Build history of the part. All positions in model axes, mm. Round coordinates to 2 decimals unless told otherwise and drop trailing zeros. Order: outer loops, then holes, each group sorted by start corner. A loop starts at its lowest first (then second) coordinate and runs counter-clockwise, first axis right, second up. Notation, with made-up numbers: (75, 55) -> (110, 55) arc R27 cw to (110, 82) -> close; hole circle Ø8 at (-2.75, 86.25). An arc over 180 degrees is marked (long way). Answer as a JSON object with one key per item and string values.
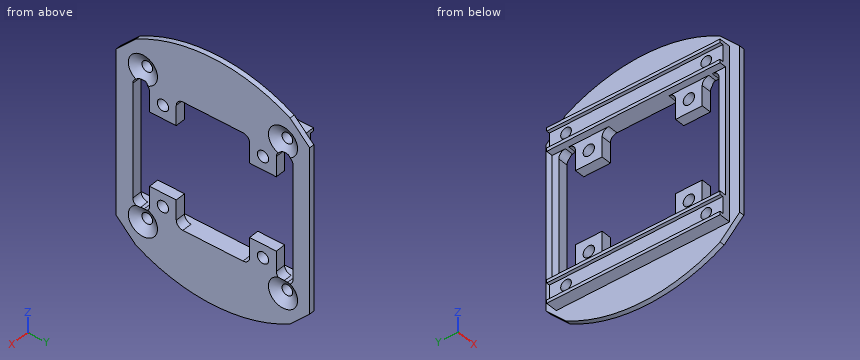
from build123d import *

# Parameters (mm, degrees)
SKETCH_1_W                  = 58
SKETCH_1_H                  = 58
SKETCH_1_R                  = 1.7
EXTRUDE_1_DEPTH             = 5
SKETCH_2_W                  = 58
SKETCH_2_H                  = 58
SKETCH_2_W_2                = 52
SKETCH_2_H_2                = 52
CUT_EXTRUDE_1_DEPTH         = 3.5
SKETCH_3_W                  = 38
SKETCH_3_H                  = 52
CUT_EXTRUDE_2_DEPTH         = 2
SKETCH_4_W                  = 5
SKETCH_4_H                  = 52
CUT_EXTRUDE_3_DEPTH         = 1
SKETCH_8_R                  = 1.6
CUT_EXTRUDE_4_DEPTH         = 2.4
PATTERN_LINEAR_1_COUNT      = 2
PATTERN_LINEAR_1_PITCH      = 45
PATTERN_LINEAR_1_COUNT_DIR2 = 2
PATTERN_LINEAR_1_PITCH_DIR2 = 42
EXTRUDE_2_DEPTH             = 1.5
SKETCH_12_R                 = 63.004873171
CUT_EXTRUDE_6_DEPTH         = 1.5
CHAMFER_2_SIZE              = 2
CHAMFER_3_SIZE              = 2
CHAMFER_5_SIZE              = 2
CHAMFER_6_SIZE              = 2


with BuildPart() as part:
    # 草图1 → 凸台-拉伸1 (new body)
    with BuildSketch(Plane(origin=(0, 0, 0), x_dir=(0, 0, -1), z_dir=(1, 0, 0))):
        Rectangle(SKETCH_1_W, SKETCH_1_H)
        with Locations((15, 15)):
            Circle(SKETCH_1_R, mode=Mode.SUBTRACT)
        with Locations(Location((-15, 15, 0), (0, 0, 180))):
            Circle(SKETCH_1_R, mode=Mode.SUBTRACT)
        with Locations((-15, -15)):
            Circle(SKETCH_1_R, mode=Mode.SUBTRACT)
        with Locations(Location((15, -15, 0), (0, 0, 180))):
            Circle(SKETCH_1_R, mode=Mode.SUBTRACT)
        with BuildLine():
            Line((-17, 24), (17, 24))
            ThreePointArc((17, 24), (18.414213562, 23.414213562), (19, 22))
            Line((19, 22), (19, 21))
            ThreePointArc((19, 21), (18.414213562, 19.585786438), (17, 19))
            Line((17, 19), (11, 19))
            Line((11, 19), (11, 11))
            Line((11, 11), (17, 11))
            ThreePointArc((17, 11), (18.414213562, 10.414213562), (19, 9))
            Line((19, 9), (19, -9))
            ThreePointArc((19, -9), (18.414213562, -10.414213562), (17, -11))
            Line((17, -11), (11, -11))
            Line((11, -11), (11, -19))
            Line((11, -19), (17, -19))
            ThreePointArc((17, -19), (18.414213562, -19.585786438), (19, -21))
            Line((19, -21), (19, -22))
            ThreePointArc((19, -22), (18.414213562, -23.414213562), (17, -24))
            Line((17, -24), (-17, -24))
            ThreePointArc((-17, -24), (-18.414213562, -23.414213562), (-19, -22))
            Line((-19, -22), (-19, -21))
            ThreePointArc((-19, -21), (-18.414213562, -19.585786438), (-17, -19))
            Line((-17, -19), (-11, -19))
            Line((-11, -19), (-11, -11))
            Line((-11, -11), (-17, -11))
            ThreePointArc((-17, -11), (-18.414213562, -10.414213562), (-19, -9))
            Line((-19, -9), (-19, 9))
            ThreePointArc((-19, 9), (-18.414213562, 10.414213562), (-17, 11))
            Line((-17, 11), (-11, 11))
            Line((-11, 11), (-11, 19))
            Line((-11, 19), (-17, 19))
            ThreePointArc((-17, 19), (-18.414213562, 19.585786438), (-19, 21))
            Line((-19, 21), (-19, 22))
            ThreePointArc((-19, 22), (-18.414213562, 23.414213562), (-17, 24))
        make_face(mode=Mode.SUBTRACT)
    extrude(amount=EXTRUDE_1_DEPTH)

    # 草图2 → 切除-拉伸1 (cut)
    with BuildSketch(Plane.ZY):
        Rectangle(SKETCH_2_W, SKETCH_2_H)
        Rectangle(SKETCH_2_W_2, SKETCH_2_H_2, mode=Mode.SUBTRACT)
    extrude(amount=-CUT_EXTRUDE_1_DEPTH, mode=Mode.SUBTRACT)

    # 草图3 → 切除-拉伸2 (cut)
    with BuildSketch(Plane.ZY):
        Rectangle(SKETCH_3_W, SKETCH_3_H)
    extrude(amount=-CUT_EXTRUDE_2_DEPTH, mode=Mode.SUBTRACT)

    # 草图4 → 切除-拉伸3 (cut)
    with BuildSketch(Plane.ZY):
        with Locations((-22.5, 0)):
            Rectangle(SKETCH_4_W, SKETCH_4_H)
        with Locations((22.5, 0)):
            Rectangle(SKETCH_4_W, SKETCH_4_H)
    extrude(amount=-CUT_EXTRUDE_3_DEPTH, mode=Mode.SUBTRACT)

    # 草图8 → 切除-拉伸4 (cut)
    with BuildSketch(Plane.ZY.offset(-1)):
        with Locations((22.5, 21)):
            Circle(SKETCH_8_R)
    cut_extrude_4 = extrude(amount=-CUT_EXTRUDE_4_DEPTH, mode=Mode.SUBTRACT)

    # 草图9 → 切除-旋转2 (revolve, cut)
    with BuildSketch(Plane.XY.offset(22.5), mode=Mode.PRIVATE) as cut_revolve_2_sk:
        Polygon((3.4, 19.4), (3.4, 21), (5, 21), (5, 16.628718708), align=None)
    cut_revolve_2 = revolve(cut_revolve_2_sk.sketch.rotate(Axis((3.417252413, 21, 22.5), (1, 0, 0)), 90), axis=Axis((3.417252413, 21, 22.5), (1, 0, 0)), mode=Mode.SUBTRACT)

    # 阵列(线性)1: 切除-拉伸4, Cut-Revolve 2 2 × 2
    with Locations(*[(0, -j * PATTERN_LINEAR_1_PITCH_DIR2, -i * PATTERN_LINEAR_1_PITCH) for i in range(PATTERN_LINEAR_1_COUNT) for j in range(PATTERN_LINEAR_1_COUNT_DIR2) if (i, j) != (0, 0)]):
        add(cut_extrude_4, mode=Mode.SUBTRACT)
        add(cut_revolve_2, mode=Mode.SUBTRACT)

    # 草图10 → 凸台-拉伸2 (add)
    with BuildSketch(Plane(origin=(5, 0, 0), x_dir=(0, 0, -1), z_dir=(1, 0, 0))):
        with BuildLine():
            Line((-29, 25.617376915), (-29, -25.617376915))
            ThreePointArc((-29, -25.617376915), (-36.5, 0), (-29, 25.617376915))
        make_face()
        with BuildLine():
            Line((29, 25.617376915), (29, -25.617376915))
            ThreePointArc((29, -25.617376915), (36.5, 0), (29, 25.617376915))
        make_face()
    extrude(amount=-EXTRUDE_2_DEPTH)

    # 草图12 → 切除-拉伸6 (cut)
    with BuildSketch(Plane(origin=(5, 0, 0), x_dir=(0, 0, -1), z_dir=(1, 0, 0))):
        Circle(SKETCH_12_R)
        with BuildLine():
            ThreePointArc((0, -46.208765402), (36.5, 0), (0, 46.208765402))
            ThreePointArc((0, 46.208765402), (-36.5, 0), (0, -46.208765402))
        make_face(mode=Mode.SUBTRACT)
    extrude(amount=-CUT_EXTRUDE_6_DEPTH, mode=Mode.SUBTRACT)

    # 倒角2
    # the kernel refuses this chamfer: 11.02112637, 2 mm, written as the material it takes off along each edge
    with BuildSketch(Plane(origin=(-15.143908505, 29, 26.619808612), x_dir=(0, 0, -1), z_dir=(1, 0, 0))) as chamfer_2_piece_1:
        with BuildLine():
            Line((CHAMFER_2_SIZE, 0), (-3.865883602, -5.865883602))
            ThreePointArc((-3.865883602, -5.865883602), (-2.160150245, -3.0422483), (0, 0))
            Line((0, 0), (CHAMFER_2_SIZE, 0))
        make_face()
    extrude(amount=38.787817011, mode=Mode.SUBTRACT)

    # 倒角3
    # the kernel refuses this chamfer: 11.02112637, 2 mm, written as the material it takes off along each edge
    with BuildSketch(Plane(origin=(-15.143908505, 29, -26.619808612), x_dir=(0, 0, 1), z_dir=(1, 0, 0))) as chamfer_3_piece_1:
        with BuildLine():
            Line((CHAMFER_3_SIZE, 0), (-3.865883602, 5.865883602))
            ThreePointArc((-3.865883602, 5.865883602), (-2.160150245, 3.0422483), (0, 0))
            Line((0, 0), (CHAMFER_3_SIZE, 0))
        make_face()
    extrude(amount=38.787817011, mode=Mode.SUBTRACT)

    # 倒角5
    # the kernel refuses this chamfer: 11.02112637, 2 mm, written as the material it takes off along each edge
    with BuildSketch(Plane(origin=(-15.143908505, -29, -26.619808612), x_dir=(0, 0, 1), z_dir=(1, 0, 0))) as chamfer_5_piece_1:
        with BuildLine():
            Line((CHAMFER_5_SIZE, 0), (-3.865883602, -5.865883602))
            ThreePointArc((-3.865883602, -5.865883602), (-2.160150245, -3.0422483), (0, 0))
            Line((0, 0), (CHAMFER_5_SIZE, 0))
        make_face()
    extrude(amount=38.787817011, mode=Mode.SUBTRACT)

    # 倒角6
    # the kernel refuses this chamfer: 11.02112637, 2 mm, written as the material it takes off along each edge
    with BuildSketch(Plane(origin=(-15.143908505, -29, 26.619808612), x_dir=(0, 0, -1), z_dir=(1, 0, 0))) as chamfer_6_piece_1:
        with BuildLine():
            Line((CHAMFER_6_SIZE, 0), (-3.865883602, 5.865883602))
            ThreePointArc((-3.865883602, 5.865883602), (-2.160150245, 3.0422483), (0, 0))
            Line((0, 0), (CHAMFER_6_SIZE, 0))
        make_face()
    extrude(amount=38.787817011, mode=Mode.SUBTRACT)


solid = part.part
1) Cut at D-D, the plane z = -15. Give the cut face in (x, y).
Checked values:
{"outline": "(2, -26) -> (3.5, -26) -> (3.5, -29) -> (5, -29) -> (5, -24) -> (2, -24) -> close; (2, -19) -> (5, -19) -> (5, -16.7) -> (2, -16.7) -> close; (2, -13.3) -> (5, -13.3) -> (5, -11) -> (2, -11) -> close; (2, 11) -> (5, 11) -> (5, 13.3) -> (2, 13.3) -> close; (2, 16.7) -> (5, 16.7) -> (5, 19) -> (2, 19) -> close; (2, 24) -> (5, 24) -> (5, 29) -> (3.5, 29) -> (3.5, 26) -> (2, 26) -> close"}
2) Cut at C-C, the plane y = -0.5. Give the cut face in (x, z), plus the area to 3 significant figures.
Checked values:
{"outline": "(0, -26) -> (3.5, -26) -> (3.5, -36.5) -> (5, -36.5) -> (5, -19) -> (0, -19) -> (0, -20) -> (1, -20) -> (1, -25) -> (0, -25) -> close; (0, 19) -> (5, 19) -> (5, 36.5) -> (3.5, 36.5) -> (3.5, 26) -> (0, 26) -> (0, 25) -> (1, 25) -> (1, 20) -> (0, 20) -> close", "area": "91.5 mm²"}
3) Flat gauge pins, fed straight in: pin 1 Ø4.5 at (y, z) = (-15, -15) entering from -X; pin 2 Ø1.1 at (x, y) = (0.5, 10) entering from +Z; pin 3 Ø2.5 at (x, y) = (2, 5) entering from -Z. Where does each tip first touch, or does it go through?
Checked values:
{"pin 1": "stops at x = 2", "pin 2": "stops at z = 26", "pin 3": "stops at z = -26"}
4) Probe L1, parallel to Z at x = 3.15, y = 15; L2, parallel to Z at x = 0.25, y = 18; L3, parallel to Y at x = 3.85, z = 15. List the from-to ranges inside material, lowest first. Write a range as from..to.
Checked values:
{"L1": "z = -26..-16.7, -13.3..-11, 11..13.3, 16.7..26", "L2": "z = -26..-25, -20..-19, 19..20, 25..26", "L3": "y = -29..-24, -19..-16.7, -13.3..-11, 11..13.3, 16.7..19, 24..29"}
5) Cut at A-A, the plane z = 6. Give the cut face in (x, y), plus the area to 3 significant figures.
Checked values:
{"outline": "(2, -26) -> (3.5, -26) -> (3.5, -29) -> (5, -29) -> (5, -24) -> (2, -24) -> close; (2, 24) -> (5, 24) -> (5, 29) -> (3.5, 29) -> (3.5, 26) -> (2, 26) -> close", "area": "21.0 mm²"}
6) Cut at B-B, the plane z = 22.5. Give the cut face in (x, y), plus the area to 3 significant figures.
Checked values:
{"outline": "(1, -26) -> (3.5, -26) -> (3.5, -29) -> (5, -29) -> (5, -25.37) -> (3.4, -22.6) -> (1, -22.6) -> close; (1, -19.4) -> (3.4, -19.4) -> (5, -16.63) -> (5, 16.63) -> (3.4, 19.4) -> (1, 19.4) -> close; (1, 22.6) -> (3.4, 22.6) -> (5, 25.37) -> (5, 29) -> (3.5, 29) -> (3.5, 26) -> (1, 26) -> close", "area": "183 mm²"}
